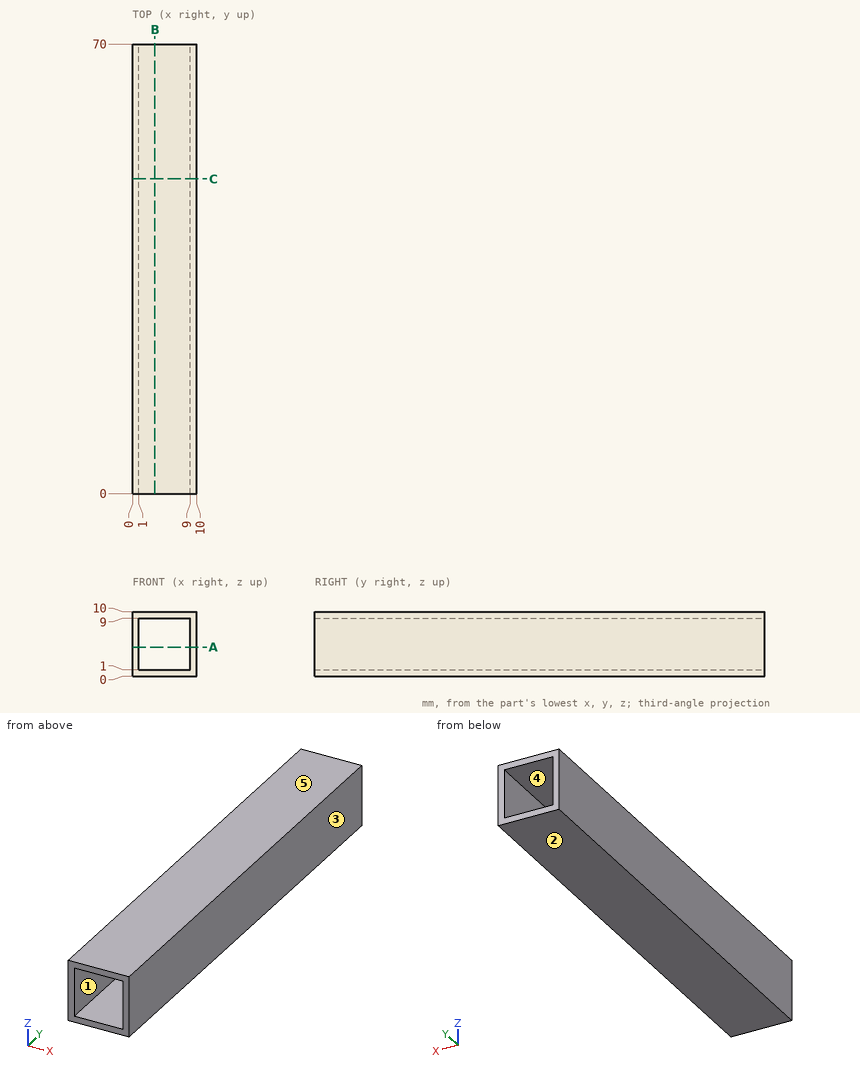
Input: dimensioned drawing with shaded views. Units: mm. Origin: part minimum x, y, z. A direction names the side the tool comes from. Give positions to 0.01 mm unless a question says otherwise; leave off trailing zeros. Write each loop counter-clockwise with the first axis right and the second up, starting at its lowest first coordinate (ties: lowest second). Pieces come first, ordered by that corner, then holes.
Q1. Set-up query: the marked faces 1 and 2. Return all of +Z, -Z, +X, -X, +Y, -Y with unobstructed straight access to the full face (end or side cutting, diameter ignored); none if empty.
Q2. Section B-B, the plane x = 3.5. Output: boundary loops of the cut face in (y, z).
Q3. Pull-direction query (X, two-part tool) for the marked faces 3, 4 and 5; classes: pulls with the +X half, pulls with the -X half, needs draft (parallel to the pull), parting line crosses it, or undercut.
Q4. Section C-C, the plane y = 49. Output: boundary loops of the cut face in (x, z).
Q5. Material intervals for probe 1 along X at (y, z) = (6, 6), sorted ascending.
Q6. Section A-A, the plane z = 4.5. Output: boundary loops of the cut face in (x, y), plus the area to 3 significant figures.
Filled in:
1. face 1: +Y, -Y
1. face 2: -Z, +X, -X, +Y, -Y
2. outline: (0, 0) - (70, 0) - (70, 1) - (0, 1) - close; (0, 9) - (70, 9) - (70, 10) - (0, 10) - close
3. face 3: pulls with the +X half
3. face 4: undercut
3. face 5: needs draft
4. outline: (0, 0) - (10, 0) - (10, 10) - (0, 10) - close; hole (1, 1) - (9, 1) - (9, 9) - (1, 9) - close
5. probe 1: x = 0 to 1, 9 to 10
6. outline: (0, 0) - (1, 0) - (1, 70) - (0, 70) - close; (9, 0) - (10, 0) - (10, 70) - (9, 70) - close
6. area: 140 mm2
